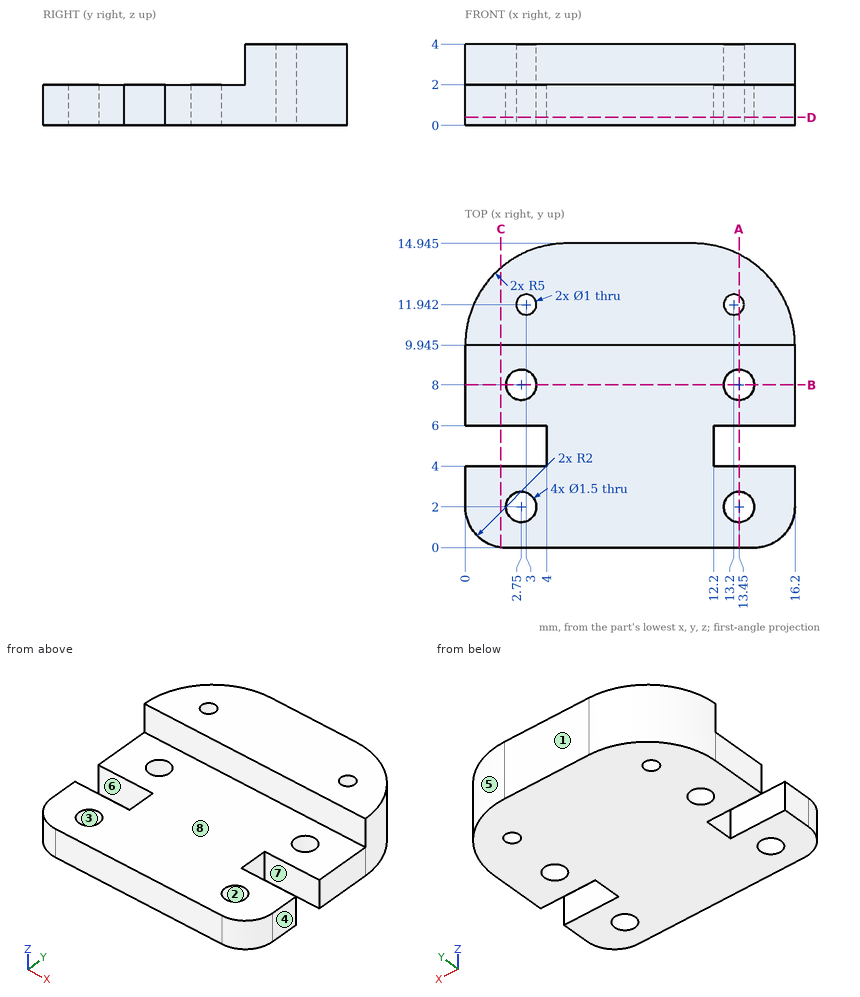
Part print with two shaded views. Sizes in mm from the minimum x, y, z corner. A direction names the side the tool comes from. Coordinates: 2 decimals unless noted, no trailing zeros. Write each loop counter-clockwise with the first axis right and the second up, starting at its lowest first coordinate (ties: lowest second). Pieces come first, ordered by that corner, then holes. Notation, with made-up numbers: (-39, -28) - (-7, -28) arc R25 cw to (-7, 10) - close; hole circle Ø4 at (45, 67). An arc over 180 degrees is marked (long way). One line per item, written item: value. Start each with the question number.
1. Tool access for the marked faces 5, 6, 7 and 8: list every direction of +Z, -Z, +X, -X, +Y, -Y with a clear straight run to the whole face (end or side of a thin tool).
2. Flat gauge pins, fed straight in: pin 1 (5 mm diameter, centred on x = 7.5, y = 10, fed in from -Z); pin 2 (0.6 mm diameter, centred on y = 4.5, z = 0.5, fed in from +X); pin 3 (1.7 mm diameter, centred on x = 2.75, y = 8, fed in from +Z); pin 4 (1 mm diameter, centred on x = 2, z = 1.5, fed in from +Y). Where does each tip first touch, or does it go through?
3. Slice it at A-A (x = 13.45). Write the cut outline in (y, z) (3 decimals), plus the area to 3 significant figures.
4. Probe line 1 (X direction, y = 8, z = 0.7); line 2 (Y direction, x = 2.25, z = 1.85); line 3 (Z direction, x = 6.25, y = 7.75). List the from-to ranges inside material, lowest first. Write a range as from..to.
5. Slice it at B-B (y = 8). Write the cut outline in (x, z).
6. Slice it at D-D (z = 0.4). Write the cut outline in (x, y) (3 decimals).
7. Mould opens along X. For the marked faces 1, 2, 3 and 4 say: released by +X, released by -X, zero draft, split by the parting line, or undercut.
8. Slice it at C-C (x = 1.75). Write the cut outline in (y, z) (3 decimals), plus the area to 3 significant figures.
Answers below:
1. face 5: +Z, -Z, +X, +Y
1. face 6: +Z, -Z, -X
1. face 7: +Z, -Z, +X
1. face 8: +Z, +X, -X, -Y
2. pin 1: stops at z = 0
2. pin 2: stops at x = 12.2
2. pin 3: stops at z = 2
2. pin 4: stops at y = 14.28
3. outline: (0, 0) - (1.25, 0) - (1.25, 2) - (0, 2) - close; (2.75, 0) - (4, 0) - (4, 2) - (2.75, 2) - close; (6, 0) - (7.25, 0) - (7.25, 2) - (6, 2) - close; (8.75, 0) - (11.509, 0) - (11.509, 4) - (9.945, 4) - (9.945, 2) - (8.75, 2) - close; (12.375, 0) - (14.41, 0) - (14.41, 4) - (12.375, 4) - close
3. area: 24.3 mm^2
4. line 1: x = 0..2, 3.5..12.7, 14.2..16.2
4. line 2: y = 0..1.44, 2.56..4, 6..7.44, 8.56..14.12
4. line 3: z = 0..2
5. outline: (0, 0) - (2, 0) - (2, 2) - (0, 2) - close; (3.5, 0) - (12.7, 0) - (12.7, 2) - (3.5, 2) - close; (14.2, 0) - (16.2, 0) - (16.2, 2) - (14.2, 2) - close
6. outline: (0, 2) arc R2 ccw to (2, 0) - (14.2, 0) arc R2 ccw to (16.2, 2) - (16.2, 4) - (12.2, 4) - (12.2, 6) - (16.2, 6) - (16.2, 9.945) arc R5 ccw to (11.2, 14.945) - (5, 14.945) arc R5 ccw to (0, 9.945) - (0, 6) - (4, 6) - (4, 4) - (0, 4) - close; hole circle Ø1.5 at (2.75, 2); hole circle Ø1.5 at (2.75, 8); hole circle Ø1 at (3, 11.942); hole circle Ø1.5 at (13.45, 2); hole circle Ø1.5 at (13.45, 8); hole circle Ø1 at (13.2, 11.942)
7. face 1: zero draft
7. face 2: undercut
7. face 3: undercut
7. face 4: released by +X
8. outline: (0.016, 0) - (4, 0) - (4, 2) - (0.016, 2) - close; (6, 0) - (13.745, 0) - (13.745, 4) - (9.945, 4) - (9.945, 2) - (6, 2) - close
8. area: 31.1 mm^2
